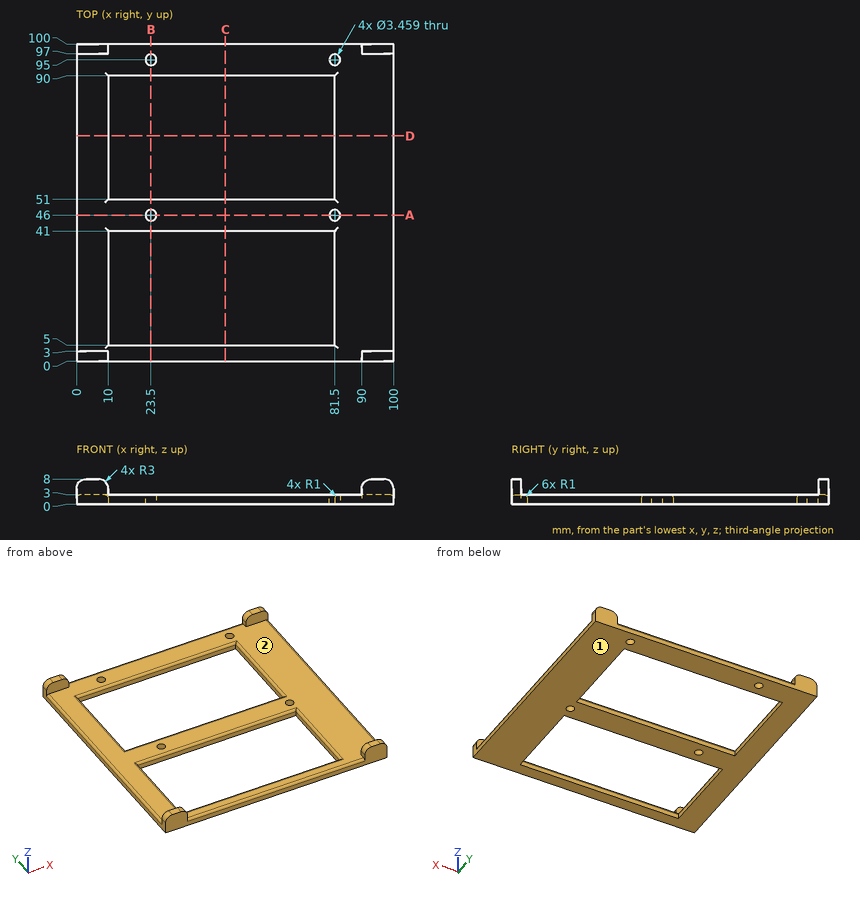
Here's the drawing with two shaded views (mm, measured from the low corner). I have some questions. Coordinates: 2 decimals unless noted, no trailing zeros. Loops run counter-clockwise (first coordinate to the right, second up) from the corner with the lowest first, then second, coordinate; pieces in that order, holes last. Notation, with made-up numbers: (49.5, 58) -> (85.5, 58) arc R16 ccw to (85.5, 83) -> close; hole circle Ø2 at (51.25, 24). An arc over 180 degrees is marked (long way). Use one line per item in the form item = value. Start each with the question number.
(1) If we section it at D-D (y = 71): Please give me the cut outline in (x, z).
(2) We'd pull the mould along Y, two halves only. Please class the marked faces 1 and 2: pulls with the +Y half, pulls with the -Y half, needs draft (parallel to the pull), parting line crosses it, or undercut.
(3) If we section it at A-A (y = 46): Please give me the cut outline in (x, z).
(4) If we section it at B-B (x = 23.5): Please give me the cut outline in (y, z).
(5) If we section it at C-C (x = 47): Please give me the cut outline in (y, z).
(6) Will this pin go through, and if not, where does the flat tip stop? pin 1 (1 mm diameter, centred on y = 15, z = 0.5, fed in from -X).
(7) Please list where these lines run through material, in increasing order: line 1 along X through (y, z) = (95, 2.15); line 2 along Y through (x, z) = (23.5, 1.55); line 3 along Y through (x, z) = (27.5, 1.5).
Verdict:
q1.outline = (0, 0) -> (10, 0) -> (10, 2) arc R1 ccw to (9, 3) -> (1, 3) arc R1 ccw to (0, 2) -> close; (81.5, 0) -> (100, 0) -> (100, 2) arc R1 ccw to (99, 3) -> (82.5, 3) arc R1 ccw to (81.5, 2) -> close
q2.face_1 = needs draft
q2.face_2 = undercut
q3.outline = (0, 0) -> (21.77, 0) -> (21.77, 3) -> (1, 3) arc R1 ccw to (0, 2) -> close; (25.23, 0) -> (79.77, 0) -> (79.77, 3) -> (25.23, 3) -> close; (83.23, 0) -> (100, 0) -> (100, 2) arc R1 ccw to (99, 3) -> (83.23, 3) -> close
q4.outline = (0, 0) -> (5, 0) -> (5, 2) arc R1 ccw to (4, 3) -> (1, 3) arc R1 ccw to (0, 2) -> close; (41, 0) -> (44.27, 0) -> (44.27, 3) -> (42, 3) arc R1 ccw to (41, 2) -> close; (47.73, 0) -> (51, 0) -> (51, 2) arc R1 ccw to (50, 3) -> (47.73, 3) -> close; (90, 0) -> (93.27, 0) -> (93.27, 3) -> (91, 3) arc R1 ccw to (90, 2) -> close; (96.73, 0) -> (100, 0) -> (100, 2) arc R1 ccw to (99, 3) -> (96.73, 3) -> close
q5.outline = (0, 0) -> (5, 0) -> (5, 2) arc R1 ccw to (4, 3) -> (1, 3) arc R1 ccw to (0, 2) -> close; (41, 0) -> (51, 0) -> (51, 2) arc R1 ccw to (50, 3) -> (42, 3) arc R1 ccw to (41, 2) -> close; (90, 0) -> (100, 0) -> (100, 2) arc R1 ccw to (99, 3) -> (91, 3) arc R1 ccw to (90, 2) -> close
q6.pin_1 = 0
q7.line_1 = 0.01 to 21.77, 25.23 to 79.77, 83.23 to 99.99
q7.line_2 = 0 to 5, 41 to 44.27, 47.73 to 51, 90 to 93.27, 96.73 to 100
q7.line_3 = 0 to 5, 41 to 51, 90 to 100
